```python
from build123d import *

# Parameters (mm, degrees)
SKETCH_1_W          = 18
SKETCH_1_H          = 18
EXTRUDE_1_DEPTH     = 3
SKETCH_2_R          = 1.65
CUT_EXTRUDE_1_DEPTH = 3
SKETCH_3_W          = 3
SKETCH_3_H          = 3
SKETCH_3_W_2        = 7.5
SKETCH_3_H_2        = 7.5
EXTRUDE_2_DEPTH     = 45
SKETCH_4_W          = 12.5
SKETCH_4_H          = 12.5
EXTRUDE_3_DEPTH     = 3
SKETCH_5_R          = 1.65
CUT_EXTRUDE_2_DEPTH = 3
CUT_EXTRUDE_3_DEPTH = 3
FILLET_1_R          = 2
FILLET_2_R          = 0.8
EXTRUDE_START       = 1
EXTRUDE_4_DEPTH     = 1
FILLET_3_R          = 1


with BuildPart() as part:
    # 草图1 → 凸台-拉伸1 (new body)
    with BuildSketch(Plane(origin=(0, 0, 0), x_dir=(1, 0, 0), z_dir=(0, 1, 0))):
        Rectangle(SKETCH_1_W, SKETCH_1_H)
    extrude(amount=EXTRUDE_1_DEPTH)

    # 草图2 → 切除-拉伸1 (cut)
    with BuildSketch(Plane(origin=(0, 3, 0), x_dir=(1, 0, 0), z_dir=(0, 1, 0))):
        with Locations(Location((-6, 6, 0), (0, 0, 270))):
            Circle(SKETCH_2_R)
        with Locations(Location((6, 6, 0), (0, 0, 270))):
            Circle(SKETCH_2_R)
        with Locations(Location((6, -6, 0), (0, 0, 270))):
            Circle(SKETCH_2_R)
        with Locations(Location((-6, -6, 0), (0, 0, 270))):
            Circle(SKETCH_2_R)
    extrude(amount=-CUT_EXTRUDE_1_DEPTH, mode=Mode.SUBTRACT)

    # 草图3 → 凸台-拉伸2 (add)
    with BuildSketch(Plane(origin=(0, 3, 0), x_dir=(1, 0, 0), z_dir=(0, 1, 0))):
        Rectangle(SKETCH_3_W, SKETCH_3_H)
        with Locations((5.25, 0)):
            Rectangle(SKETCH_3_W_2, SKETCH_3_H)
        with Locations((0, -5.25)):
            Rectangle(SKETCH_3_W, SKETCH_3_H_2)
    extrude(amount=EXTRUDE_2_DEPTH)

    # 草图4 → 凸台-拉伸3 (add)
    with BuildSketch(Plane(origin=(0, 48, 0), x_dir=(1, 0, 0), z_dir=(0, 1, 0))):
        with Locations((4.75, -4.75)):
            Rectangle(SKETCH_4_W, SKETCH_4_H)
    extrude(amount=EXTRUDE_3_DEPTH)

    # 草图5 → 切除-拉伸2 (cut)
    with BuildSketch(Plane(origin=(0, 51, 0), x_dir=(1, 0, 0), z_dir=(0, 1, 0))):
        with Locations(Location((5, -5, 0), (0, 0, 270))):
            Circle(SKETCH_5_R)
    extrude(amount=-CUT_EXTRUDE_2_DEPTH, mode=Mode.SUBTRACT)

    # 草图6 → 切除-拉伸3 (cut)
    with BuildSketch(Plane(origin=(0, 3, 0), x_dir=(1, 0, 0), z_dir=(0, 1, 0))):
        Polygon((-9, 9), (-9, 0.329900852), (-0.974802815, 9), align=None)
    extrude(amount=-CUT_EXTRUDE_3_DEPTH, mode=Mode.SUBTRACT)

    # 圆角1
    fillet_1_edges = [part.edges().sort_by_distance(p)[0] for p in [
        (-9, 1.5, 9),
        (9, 1.5, 9),
        (9, 1.5, -9),
        (-1.5, 49.5, 11),
        (11, 49.5, 11),
        (11, 49.5, -1.5),
        (1.5, 25.5, 1.5),
        (-1.5, 27, -1.5),
    ]]
    fillet(fillet_1_edges, radius=FILLET_1_R)

    # 圆角2
    fillet_2_edges = [part.edges().sort_by_distance(p)[0] for p in [
        (2.085786438, 3, 2.085786438),
        (-0.914213562, 3, -0.914213562),
        (1.5, 3, 6.25),
        (-1.5, 3, 4.75),
        (6.25, 3, 1.5),
        (4.75, 3, -1.5),
    ]]
    fillet(fillet_2_edges, radius=FILLET_2_R)

    # 草图7 → 凸台-拉伸4 (add)
    with BuildSketch(Plane(origin=(0, 51, 0), x_dir=(1, 0, 0), z_dir=(0, 1, 0)).offset(EXTRUDE_START)):
        with BuildLine():
            Line((0.5, -11), (0.5, -0.5))
            Line((0.5, -0.5), (11, -0.5))
            ThreePointArc((11, -0.5), (10.414213562, 0.914213562), (9, 1.5))
            Line((9, 1.5), (0.5, 1.5))
            ThreePointArc((0.5, 1.5), (-0.914213562, 0.914213562), (-1.5, -0.5))
            Line((-1.5, -0.5), (-1.5, -9))
            ThreePointArc((-1.5, -9), (-0.914213562, -10.414213562), (0.5, -11))
        make_face()
    extrude(amount=-EXTRUDE_4_DEPTH)

    # 圆角3
    fillet_3_edges = [part.edges().sort_by_distance(p)[0] for p in [
        (0.5, 51.5, 0.5),
    ]]
    fillet(fillet_3_edges, radius=FILLET_3_R)


solid = part.part
```
Here's how the part is built. I have some questions about the finished solid (model axes, mm). A direction names the side the tool comes from. Give positions to 0.01 mm unless a question says otherwise; leave off trailing zeros. Order: outer loops, then holes, each group sorted by start corner. A loop starts at its lowest first (then second) coordinate and runs counter-clockwise, first axis right, second up. Notation, with made-up numbers: M 43,25 L 57,25 A21 ccw 57,42 Z; hole C 43,-2.75 d8. An arc over 180 degrees is marked long. Use a Markdown table: item, result. Add a question column.
1. If we mould it in two halves opening along X, with no side actions, what happens to faces 5 (the cylindrical face through (5, 1.52, -7.31)), 6 (the flat face through (6.2, 51.5, 0.5)), 7 (the cylindrical face through (-0.9, 28.24, -0.93))? For each: +X half, -X half, draft (parallel to the pull), parting line (faces both ways), or undercut.
2. For pin 1 Ø0.8 at (y, z) = (51.5, 6) entering from +X; pin 2 Ø7 at (y, z) = (13, 1.5) entering from +X; pin 3 Ø1.5 at (x, z) = (1.5, 4.5) entering from +Y, each with a flat end and sliding along its axis, tell me the tip position at first contact or that it passes through.
3. Suppose I cut it at C-C (y = 19). List the corners of the cut face in (x, z) for me, and give its area (3 significant figures).
4. Suppose I cut it at A-A (z = 5.25). List the corners of the cut face in (x, y) for me, and give its area (3 significant figures).
5. On a 3-axis mill with a long thin cutter (end or side, diameter ignored), from which of +Z, -Z, +X, -X, +Y, -Y can I reach the whole of each face in a straight line? I mean faces 1 (the flat face through (6, 3, 4)), 2 (the cylindrical face through (4, 49.52, 3.69)), 3 (the flat face through (-2, 3, -2)), 4 (the flat face through (0, 19, 9)). Say none if no direction works.
6. Suppose I cut it at B-B (x = -6). List the corners of the cut face in (y, z) for me, and give its area (3 significant figures).
7. Suppose I cut it at D-D (x = 5). List the corners of the cut face in (y, z) for me, and give its area (3 significant figures).
8. I need wall thicknesses on probe 1 along X at (y, z) = (2.15, 6); probe 2 along Y at (x, z) = (3, 4.5); probe 3 along Y at (x, z) = (10.25, 8.5). Which ranges of each line are inside material? Lowest first, please. Write a range as from..to.
Results list:
| question | item | result |
|---|---|---|
| 1 | face 5 | undercut |
| 1 | face 6 | draft |
| 1 | face 7 | -X half |
| 2 | pin 1 | stops at x = 0.5 |
| 2 | pin 2 | stops at x = 9 |
| 2 | pin 3 | stops at y = 51 |
| 3 | outline | M -1.5,0.5 A2 ccw 0.5,-1.5 L 9,-1.5 L 9,1.5 L 3.5,1.5 A2 cw 1.5,3.5 L 1.5,9 L -1.5,9 Z |
| 3 | area | 54.0 mm² |
| 4 | outline | M -9,0 L -7.47,0 L -7.47,3 L -9,3 Z; M -4.53,0 L 4.53,0 L 4.53,3 L 2.3,3 A0.8 cw 1.5,3.8 L 1.5,48 L 3.37,48 L 3.37,51 L 0.5,51 L 0.5,52 L -1.5,52 L -1.5,3.8 A0.8 cw -2.3,3 L -4.53,3 Z; M 6.63,48 L 11,48 L 11,51 L 6.63,51 Z; M 7.47,0 L 9,0 L 9,3 L 7.47,3 Z |
| 4 | area | 201 mm² |
| 5 | face 1 | +Z, +X |
| 5 | face 2 | +Y |
| 5 | face 3 | -Z, -X, +Y |
| 5 | face 4 | +Z, +X, -X, -Y |
| 6 | outline | M 0,-3.57 L 3,-3.57 L 3,4.35 L 0,4.35 Z; M 0,7.65 L 3,7.65 L 3,9 L 0,9 Z |
| 6 | area | 27.8 mm² |
| 7 | outline | M 0,-9 L 3,-9 L 3,-7.31 L 0,-7.31 Z; M 0,-4.69 L 3,-4.69 L 3,-2.3 A0.8 cw 3.8,-1.5 L 52,-1.5 L 52,0.5 L 51,0.5 L 51,3.35 L 48,3.35 L 48,1.5 L 3.8,1.5 A0.8 cw 3,2.3 L 3,4.69 L 0,4.69 Z; M 0,7.31 L 3,7.31 L 3,9 L 0,9 Z; M 48,6.65 L 51,6.65 L 51,11 L 48,11 Z |
| 7 | area | 203 mm² |
| 8 | probe 1 | x = -9..-7.65, -4.35..4.35, 7.65..9 |
| 8 | probe 2 | y = 0..3, 48..51 |
| 8 | probe 3 | y = 48..51 |
